from build123d import *

# Parameters (mm, degrees)
SKETCH1_W           = 138.84292961
SKETCH1_H           = 131.475201729
BOSS_EXTRUDE1_DEPTH = 8
BOSS_EXTRUDE2_REACH = 234.154
SKETCH3_W           = 138.84292961
SKETCH3_H           = 5
CUT_EXTRUDE1_REACH  = 235.486
SKETCH5_R           = 2
CUT_EXTRUDE2_DEPTH  = 234.486082153


with BuildPart() as part:
    # Sketch1 → Boss-Extrude1 (new body)
    with BuildSketch(Plane.XY):
        with Locations((121.747366115, -65.737600865)):
            Rectangle(SKETCH1_W, SKETCH1_H)
    extrude(amount=-BOSS_EXTRUDE1_DEPTH)

    # Boss-Extrude2: up to this plane
    boss_extrude2_end = Plane(origin=(52.32590131, -131.475201729, -26.162950407), z_dir=(-0.001800589328445012, 0, 0.9999983789377211))
    # Sketch3 → Boss-Extrude2 (add, up to the surface)
    with BuildSketch(Plane.XY, mode=Mode.PRIVATE) as boss_extrude2_sk1:
        with Locations((121.747366115, -2.5)):
            Rectangle(SKETCH3_W, SKETCH3_H)
    boss_extrude2_tool1 = split(extrude(boss_extrude2_sk1.sketch, amount=-BOSS_EXTRUDE2_REACH, mode=Mode.PRIVATE), bisect_by=boss_extrude2_end, keep=Keep.BOTH, mode=Mode.PRIVATE)
    add(boss_extrude2_tool1.solids().sort_by_distance((121.747366, -2.5, 0))[0])
    # Sketch3 → Boss-Extrude2 (add, up to the surface)
    with BuildSketch(Plane.XY, mode=Mode.PRIVATE) as boss_extrude2_sk2:
        with Locations((121.747366115, -128.975201729)):
            Rectangle(SKETCH3_W, SKETCH3_H)
    boss_extrude2_tool2 = split(extrude(boss_extrude2_sk2.sketch, amount=-BOSS_EXTRUDE2_REACH, mode=Mode.PRIVATE), bisect_by=boss_extrude2_end, keep=Keep.BOTH, mode=Mode.PRIVATE)
    add(boss_extrude2_tool2.solids().sort_by_distance((121.747366, -128.975202, 0))[0])

    # Sketch4 → Cut-Extrude1 (cut, up to next)
    with BuildSketch(Plane.XZ.offset(131.475201729), mode=Mode.PRIVATE) as cut_extrude1_sk1:
        Polygon((135.612712051, -26.012984821), (128.698898599, -14.037908649), (114.842492139, -14.037908649), (108.015470014, -26.062676201), align=None)
    cut_extrude1_tool1 = extrude(cut_extrude1_sk1.sketch, amount=-CUT_EXTRUDE1_REACH, mode=Mode.PRIVATE) & part.part
    add(cut_extrude1_tool1.solids().sort_by_distance((121.790009, -131.475202, -20.700826))[0], mode=Mode.SUBTRACT)

    # Sketch5 → Cut-Extrude2 (cut, through all)
    with BuildSketch(Plane.XZ.offset(131.475201729)):
        with Locations(Location((86.267027305, -13.435028843, 0), (0, 0, 270))):
            Circle(SKETCH5_R)
        with Locations(Location((156.977705423, -13.435028843, 0), (0, 0, 270))):
            Circle(SKETCH5_R)
    extrude(amount=-CUT_EXTRUDE2_DEPTH, mode=Mode.SUBTRACT)


solid = part.part
Geometry: final body of the model. Coordinates: model frame, mm. A direction names the side the tool comes from. Coordinates: 2 decimals unless noted, no trailing zeros. Write each loop counter-clockwise with the first axis right and the second up, starting at its lowest first coordinate (ties: lowest second). Pieces come first, ordered by that corner, then holes. Notation, with made-up numbers: (3, 40) - (20, 40) arc R31 cw to (20, 77) - close; hole circle Ø5 at (20.25, -3.5). An arc over 180 degrees is marked (long way). Return JSON: item names as keys, results as strings.
Item 1: Line query: L1, parallel to Y at x = 103, z = -10.75; L2, parallel to Z at x = 122, y = -84.5; L3, parallel to Y at x = 133, z = -24. Output: solid intervals per line, ascending.
Completed:
{"L1": "y = -131.48 to -126.48, -5 to 0", "L2": "z = -8 to 0", "L3": "y = -5 to 0"}
Item 2: Section query B-B (x = 119). Output: boundary loops of the cut face in (y, z), and give its area (3 significant figures).
Completed:
{"outline": "(-131.48, -14.04) - (-126.48, -14.04) - (-126.48, -8) - (-5, -8) - (-5, -26.04) - (0, -26.04) - (0, 0) - (-131.48, 0) - close", "area": "1,170 mm2"}
Item 3: Section query A-A (z = -18.5). Output: boundary loops of the cut face in (x, y).
Completed:
{"outline": "(52.33, -131.48) - (112.31, -131.48) - (112.31, -126.48) - (52.33, -126.48) - close; (52.33, -5) - (191.17, -5) - (191.17, 0) - (52.33, 0) - close; (131.28, -131.48) - (191.17, -131.48) - (191.17, -126.48) - (131.28, -126.48) - close"}
Item 4: Reachability of faces 1 (the face through (155.203, -2.535, -14.358)), 2 (the face through (121, -5, -17)), 3 (the face through (111.477, -129.01, -19.966)) from +Z, -Z, +X, -X, +Y, -Y: full face, straight path, thin tool, end or side. Return the list, or none.
Completed:
{"face 1": "+Y, -Y", "face 2": "-Z, +X, -X", "face 3": "-Z, -Y"}
Item 5: Pin query (flat end, axial travel): pin 1 Ø2.5 at (x, z) = (156.98, -13.44) entering from +Y; pin 2 Ø12 at (y, z) = (-57.5, -11.5) entering from +X; pin 3 Ø5 at (x, y) = (140.5, -40.5) entering from -Z; pin 4 Ø2.5 at (x, y) = (122, -128.5) entering from -Z. Return the tip coordinate at first contact, or that it passes through.
Completed:
{"pin 1": "passes through", "pin 2": "stops at x = 191.17", "pin 3": "stops at z = -8", "pin 4": "stops at z = -14.04"}
Item 6: Pull-direction query (X, two-part tool) for faces 4 (the face through (52.326, -66, -5)), 5 (the face through (121, -65, 0)), 6 (the face through (155.203, -129.01, -14.358)), 7 (the face through (132.2, -129, -20.1)); classes: +X half, -X half, draft (parallel to the pull), parting line (faces both ways), or undercut.
Completed:
{"face 4": "-X half", "face 5": "draft", "face 6": "undercut", "face 7": "undercut"}
Item 7: Section query C-C (y = -21). Output: boundary loops of the cut face in (x, z), and give its area (3 significant figures).
Completed:
{"outline": "(52.33, -8) - (191.17, -8) - (191.17, 0) - (52.33, 0) - close", "area": "1,110 mm2"}
Item 8: Section query D-D (x = 161). Output: boundary loops of the cut face in (y, z).
Completed:
{"outline": "(-131.48, -25.97) - (-126.48, -25.97) - (-126.48, -8) - (-5, -8) - (-5, -25.97) - (0, -25.97) - (0, 0) - (-131.48, 0) - close"}
